Source: CAD feature listing. Evaluate the final solid. Frame: model axes, mm. A direction names the side the tool comes from. Coordinates: 2 decimals unless noted, no trailing zeros. Write each loop counter-clockwise with the first axis right and the second up, starting at its lowest first coordinate (ties: lowest second). Pieces come first, ordered by that corner, then holes. Notation, with made-up numbers: M 73,69 L 116,69 A18 cw 116,88 Z; hole C 52.5,22 d10. An arc over 180 degrees is marked long. Answer as CSV lines item,"result". Start each with the question number.
1. Section D-D on z = -13.75. Return the cut outline in (x, y), plus the area to 3 significant figures.
2. Section A-A on x = 0. Count the separate pieces of the cut face and the enclosed holes in it, plus the area to 3 significant figures.
3. Contact query for flat-ended pins moving along their axis: pin 1 Ø8 at (y, z) = (2.5, -8.5) entering from +X; pin 2 Ø8 at (x, z) = (-7, -8.5) entering from -Y; pin 3 Ø8 at (x, z) = (-6.5, -23) entering from -Y; pin 4 Ø9.5 at (x, y) = (0, 0) entering from +Z. Output: stop coordinate, or through.
4. Line query: probe 1 along Y at (x, z) = (0, -22.1); probe 2 along Z at (x, y) = (-9, -18); probe 3 along X at (y, z) = (-1, -2). Output: solid intervals per line, ascending. Write a range as [from, to].
5. Section C-C on x = -11. Return the cut outline in (y, z), plus the area to 3 significant figures.
6. Mould query, pull axis X, two halves, no side actions, for faces 1 (the face through (-9.129, -9.256, -23.465)), 2 (the face through (17.2, 1.5, -19.5)), 3 (the face through (0, -7, -24)), 4 (the face through (6.31, 20.03, -0.74)). Classes: pulls with the +X half, pulls with the -X half, needs draft (parallel to the pull), parting line crosses it, or undercut.
7. Reachability of faces 5 (the face through (-9.256, 9.129, -23.465)), 6 (the face through (0, 7, -24)), 7 (the face through (9.256, -9.129, -23.465)) from +Z, -Z, +X, -X, +Y, -Y: full face, straight path, thin tool, end or side. Return the list, or none.
```python
from build123d import *

# Parameters (mm, degrees)
SKETCH2_R                                           = 6
CUT_EXTRUDE1_DEPTH                                  = 27
CBORE_FOR_M4_HEX_SOCKET_HEAD_CAP_SCREW1_D           = 4
CBORE_FOR_M4_HEX_SOCKET_HEAD_CAP_SCREW1_CBORE_D     = 8
CBORE_FOR_M4_HEX_SOCKET_HEAD_CAP_SCREW1_CBORE_DEPTH = 5
CHAMFER1_SIZE                                       = 0.5


with BuildPart() as part:
    # Sketch1 → Revolve1 (revolve)
    with BuildSketch(Plane(origin=(0, 0, 0), x_dir=(0, 0, -1), z_dir=(1, 0, 0))):
        Polygon((0, 0), (26, 0), (26, 13), (21, 13), (21, 21), (19.5, 21), (19.5, 16.9), (1.5, 16.9), (1.5, 21), (0, 21), align=None)
    revolve(axis=Axis((0, 0, 0), (0, 0, -1)))

    # Sketch2 → Cut-Extrude1 (cut, through all)
    with BuildSketch(Plane(origin=(0, 0, -26), x_dir=(-1, 0, 0), z_dir=(0, 0, -1))):
        Circle(SKETCH2_R)
    extrude(amount=-CUT_EXTRUDE1_DEPTH, mode=Mode.SUBTRACT)

    # CBORE for M4 Hex Socket Head Cap Screw1 (through all)
    with Locations(Plane(origin=(0, 0, -26), x_dir=(-1, 0, 0), z_dir=(0, 0, -1))):
        with Locations((0, 11), (11, 0), (0, -11), (-11, 0)):
            CounterBoreHole(CBORE_FOR_M4_HEX_SOCKET_HEAD_CAP_SCREW1_D / 2, CBORE_FOR_M4_HEX_SOCKET_HEAD_CAP_SCREW1_CBORE_D / 2, CBORE_FOR_M4_HEX_SOCKET_HEAD_CAP_SCREW1_CBORE_DEPTH)

    # Chamfer1
    chamfer1_edges = [part.edges().sort_by_distance(p)[0] for p in [
        (6, 0, 0),
    ]]
    chamfer(chamfer1_edges, length=CHAMFER1_SIZE)


solid = part.part
```
Values:
1,outline,"C 0,0 d33.8; hole C -11,0 d4; hole C 0,0 d12; hole C 0,-11 d4; hole C 0,11 d4; hole C 11,0 d4"
1,area,"734 mm²"
2,separate pieces,"4"
2,enclosed holes,"0"
2,area,"324 mm²"
3,pin 1,"x = 16.9"
3,pin 2,"y = -16.63"
3,pin 3,"y = -20.78"
3,pin 4,"through"
4,probe 1,"[-7, -6], [6, 7]"
4,probe 2,"[-21, -19.5], [-1.5, 0]"
4,probe 3,"[-16.87, -12.73], [-9.27, -5.92], [5.92, 9.27], [12.73, 16.87]"
5,outline,"M -17.89,-21 L -6.93,-21 L -6.93,-26 L -4,-26 L -4,-21 L -2,-21 L -2,0 L -17.89,0 L -17.89,-1.5 L -12.83,-1.5 L -12.83,-19.5 L -17.89,-19.5 Z; M 2,-21 L 4,-21 L 4,-26 L 6.93,-26 L 6.93,-21 L 17.89,-21 L 17.89,-19.5 L 12.83,-19.5 L 12.83,-1.5 L 17.89,-1.5 L 17.89,0 L 2,0 Z"
5,area,"514 mm²"
6,face 1,"pulls with the -X half"
6,face 2,"needs draft"
6,face 3,"undercut"
6,face 4,"parting line crosses it"
7,face 5,"-Z, -X, +Y"
7,face 6,"-Z"
7,face 7,"-Z, +X, -Y"
